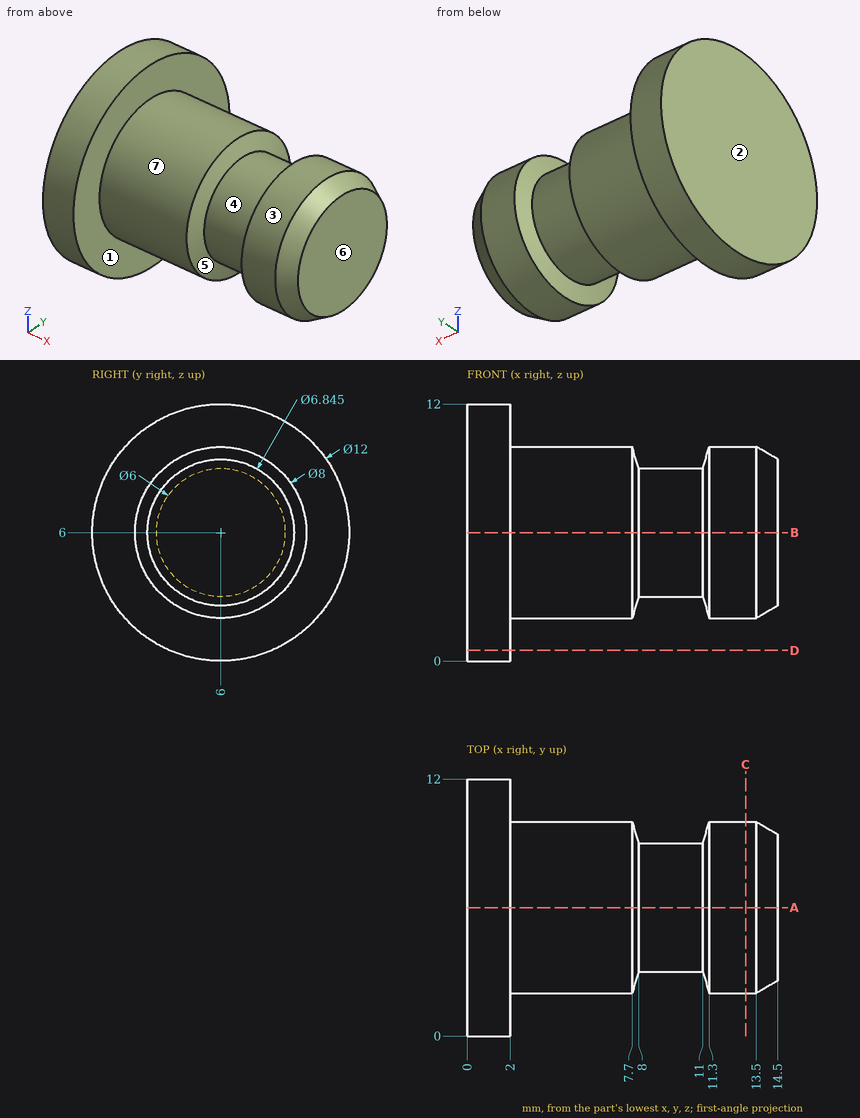
Input: dimensioned drawing with shaded views. Units: mm. Origin: part minimum x, y, z. A direction names the side the tool comes from. Give positions to 0.01 mm unless a question says otherwise; leave off trailing zeros. Write each loop counter-clockwise with the first axis right and the second up, starting at its lowest first coordinate (ties: lowest second). Pieces come first, ordered by that corner, then holes. Notation, with made-up numbers: (-12, -11) -> (10, -11) arc R24 ccw to (10, 21) -> close; hole circle Ø11 at (-7.5, -39). An arc over 180 degrees is marked (long way). Return JSON: item names as keys, results as strings. Group by question number.
1. Section A-A, the plane y = 6. Output: boundary loops of the cut face in (x, z).
2. Section D-D, the plane z = 0.5. Output: boundary loops of the cut face in (x, y).
3. Mould query, pull axis X, two halves, no side actions, for the marked faces 1, 2, 3 and 4. Classes: +X half, -X half, draft (parallel to the pull), parting line (faces both ways), or undercut.
4. Pin query (flat end, axial travel): pin 1 Ø6 at (x, y) = (12.5, 8.5) entering from -Z; pin 2 Ø3 at (x, z) = (7.5, 9) entering from -Y; pin 3 Ø1 at (x, z) = (8.5, 4) entering from -Y; pin 4 Ø1 at (x, z) = (9, 1.5) entering from +Y. Return the tip coordinate at first contact, or that it passes through.
5. Access query for the marked faces 5, 6 and 7. Directions: +Z, -Z, +X, -X, +Y, -Y. A direction counts if a zero-diameter tool reaches every point of the face in a straight line with its end or side. Return the directions, or none.
6. Material intervals for line 1 (X direction, y = 8.75, z = 3.75) (1 decimal); line 2 (X direction, y = 8.25, z = 1.75); line 3 (Z direction, x = 7, y = 6), sorted ascending. Write a range as from..to.
7. Section C-C, the plane x = 13. Output: boundary loops of the cut face in (y, z).
Determined:
{
 "1": {"outline": "(0, 0) -> (2, 0) -> (2, 2) -> (7.7, 2) -> (8, 3) -> (11, 3) -> (11.3, 2) -> (13.5, 2) -> (14.5, 2.58) -> (14.5, 9.42) -> (13.5, 10) -> (11.3, 10) -> (11, 9) -> (8, 9) -> (7.7, 10) -> (2, 10) -> (2, 12) -> (0, 12) -> close"},
 "2": {"outline": "(0, 3.6) -> (2, 3.6) -> (2, 8.4) -> (0, 8.4) -> close"},
 "3": {"face 1": "+X half", "face 2": "-X half", "face 3": "draft", "face 4": "undercut"},
 "4": {"pin 1": "stops at z = 2", "pin 2": "stops at y = 2.29", "pin 3": "stops at y = 3.4", "pin 4": "passes through"},
 "5": {"face 5": "none", "face 6": "+Z, -Z, +X, +Y, -Y", "face 7": "+X"},
 "6": {"line 1": "x = 0..7.8, 11.2..14.3", "line 2": "x = 0..2", "line 3": "z = 2..10"},
 "7": {"outline": "circle Ø8 at (6, 6)"}
}
